For this review, take the finished solid that the model builds, in its own axes (mm). Face numbers are marked on the shaded views. A direction names the side the tool comes from. Coordinates: 2 decimals unless noted, no trailing zeros. Write each loop counter-clockwise with the first axis right and the second up, starting at its lowest first coordinate (ties: lowest second). Pieces come first, ordered by that corner, then holes.
1) To check wall thickness, follow line 1 along X through (y, z) = (-63, 0); line 2 along Z through (x, y) = (23, -10.5). State the ranges of each line that lie inside material, in increasing order.
2) For the marked faces 1, 2 and 3, list the 3-axis set-ups (+Z, -Z, +X, -X, +Y, -Y) from which the entire face can be reached by the end or side of a thin tool; tool diameter is ignored.
3) We need section A-A on z = 54.5. Write out the cut boundary in (x, y).
4) Insertion check: P1, Ø3, axis at x = 0, y = 53, coming from the -Z side; P2, Ø1, axis at y = 11.5, z = 33, coming from the +X side; P3, Ø1, axis at y = -54.5, z = 19.5, coming from the +X side. Each pin has a flat end and moves straight along its axis. Give the tip position at first contact, or say it passes through.
5) Mouldability with a two-part tool opening along Z and no side actions: class the marked faces 4, 5, 6 and 7 as pulls with the +Z half, pulls with the -Z half, needs draft (parallel to the pull), parting line crosses it, or undercut.
Autodesk Inventor part; units mm, degrees
ref_plane "YZ Plane" through (0, 0, 0) normal (1, 0, 0) x (0, 1, 0)
ref_plane "XZ Plane" through (0, 0, 0) normal (0, 1, 0) x (-1, 0, 0)
ref_plane "XY Plane" through (0, 0, 0) normal (0, 0, 1) x (1, 0, 0)
sketch "Sketch_1" plane through (0, 0, 0) normal (1, 0, 0) x (0, 1, 0)
  line L0 (61.0702, 0) -> (61.0702, -13.6667)
  line L1 (61.0702, -13.6667) -> (58.5831, -20.5)
  line L2 (58.5831, -20.5) -> (40.0529, -20.5)
  line L3 (40.0529, -20.5) -> (38.848, -17.1896)
  line L4 (38.848, -17.1896) -> (38.848, -13.6667)
  line L5 (-38.848, -13.6667) -> (-38.848, -17.1896)
  line L6 (-38.848, -17.1896) -> (-40.0529, -20.5)
  line L7 (-40.0529, -20.5) -> (-58.5831, -20.5)
  line L8 (-58.5831, -20.5) -> (-61.0702, -13.6667)
  line L9 (-61.0702, -13.6667) -> (-61.0702, 0)
  line L10 (-61.0702, 0) -> (61.0702, 0)
  line L11 (-40.0529, -20.5) -> (0, -20.5) construction
  line L12 (0, -20.5) -> (0, -30.1874) construction
  line L13 (-59.3111, -20.5) -> (-42.0529, -20.5)
  line L14 (-42.0529, -20.5) -> (-42.0529, -18.5)
  line L15 (-42.0529, -18.5) -> (-59.3111, -18.5)
  line L16 (-59.3111, -18.5) -> (-59.3111, -20.5)
  line L17 (42.0529, -20.5) -> (59.3111, -20.5)
  line L18 (59.3111, -20.5) -> (59.3111, -18.5)
  line L19 (59.3111, -18.5) -> (42.0529, -18.5)
  line L20 (42.0529, -18.5) -> (42.0529, -20.5)
  line L21 (-38.848, -13.6667) -> (38.848, -13.6667)
  point P0 (0, 0)
  point P1 (0, 0)
  point P2 (-49.318, -20.5)
  point P3 (50.682, -20.5)
  point P4 (0, 0)
  dimension "dimE" = 41
  dimension "d22" = 20.5
  dimension "d23" = 6.8333
  dimension "d24" = 20
  dimension "d27" = 22.2222
  dimension "d28" = 22.2222
  dimension "d52" = 20
  dimension "d53" = 2
  dimension "d54" = 2
  dimension "d55" = 2
  dimension "dimZ" = 100
revolve "Revolution1" add sketch "Sketch_1" angle 360 about axis through (0, -61.0702, 0) along (0, 1, 0) contours L0 L1 L19 L20 L2 L3 L4 L21 L5 L6 L7 L14 L15 L8 L9 L10 | L1 L2 L20 L19 | L15 L14 L7 L8 | L8 L13 L16
sketch "Sketch11" plane through (0, 0, 0) normal (0, 0, 1) x (1, 0, 0)
  line L0 (-23.848, 23.848) -> (23.848, 23.848)
  line L1 (23.848, 23.848) -> (23.848, -23.848)
  line L2 (23.848, -23.848) -> (-23.848, -23.848)
  line L3 (-23.848, -23.848) -> (-23.848, 23.848)
  line L4 (23.848, -23.848) -> (-23.848, 23.848)
  line L5 (17.1896, 38.848) -> (-17.1896, 38.848)
  point P0 (0, 0)
  point P1 (0, 0)
  point P2 (0, 0)
  dimension "d71" = 15
extrude "Extrusion6" add sketch "Sketch11" along normal blind 34
sketch "Sketch_2" plane through (0, 0, 0) normal (1, 0, 0) x (0, 1, 0)
  line L0 (0, 34) -> (23.848, 34)
  line L1 (23.848, 34) -> (23.848, 56.2222)
  line L2 (23.848, 56.2222) -> (0, 56.2222)
  line L3 (0, 56.2222) -> (0, 34)
  line L4 (0, 56.2222) -> (34.9591, 56.2222)
  line L5 (34.9591, 56.2222) -> (34.9591, 129)
  line L6 (34.9591, 129) -> (0, 129)
  line L7 (0, 129) -> (0, 56.2222)
  line L8 (-33.3229, 0) -> (54.4515, 0)
  line L9 (-90.3, 0) -> (90.3, 0)
  line L10 (0, -319.9275) -> (0, 424.6014)
  point P0 (10.5643, 0)
  dimension "d67" = 22.2222
  dimension "d68" = 129
  dimension "d70" = 11.1111
revolve "Revolution2" add sketch "Sketch_2" angle 360 about axis through (0, 0, 129) along (0, 0, -1)
fillet "Fillet1" radius 6.7 4 edges at (-23.848, 23.848, 17) (-23.848, -23.848, 17) (23.848, -23.848, 17) (23.848, 23.848, 17)
sketch "Sketch_7" plane through (0, 0, 0) normal (1, 0, 0) x (0, 1, 0)
  line L0 (-64.5, 12.5) -> (64.5, 12.5)
  line L1 (48.5126, 0) -> (-48.5126, 0)
  line L2 (-64.5, 12.5) -> (-64.5, 10)
  line L3 (-64.5, 10) -> (64.5, 10)
  line L4 (64.5, 10) -> (64.5, 12.5)
  line L5 (0, 0.4963) -> (0, 17.9963)
  point P0 (0, 0)
  point P1 (0, 0)
  point P2 (0, 10)
  point P3 (0, 0)
  dimension "dimH" = 129
  dimension "dimD" = 20
  dimension "dimD2" = 25
revolve "Revolution3" add sketch "Sketch_7" angle 360 about axis through (0, 48.5126, 0) along (0, -1, 0)
extrude "Extrusion8" cut sketch "Sketch_1" along normal mid plane 2.7333 contours L18 L17 L1 | L1 L2 L20 L19 | L15 L14 L7 L8 | L8 L13 L16
pattern_circular "Circular Pattern1" count 6 over 360 about axis through (0, 32.25, 0) along (0, -1, 0) of "Extrusion8"
equation "\"d23\" = 0.333333 * d22"
equation "\"d27\" = 0.222222 * dimZ"
equation "\"d28\" = d27"
equation "\"d35\" = 0.1 * dimC"
equation "\"d47\" = 0.0666667 * dimE"
properties part number "DIAPHRAGM VALVE PNEUMATIC GLUED DN15" material "PVC"
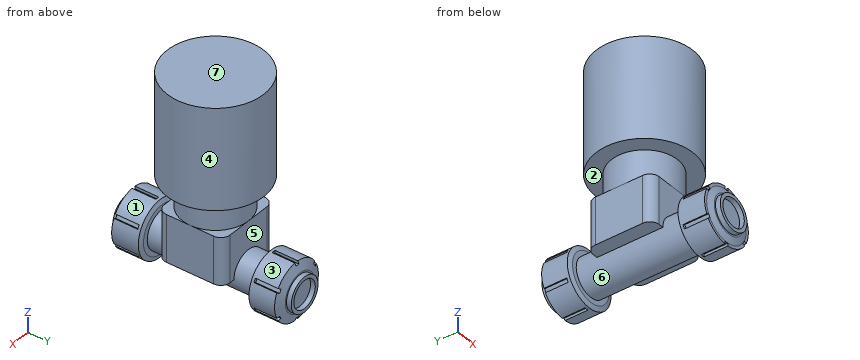
Result:
1. line 1: x = -12.5 to -10, 10 to 12.5
1. line 2: z = 0 to 34, 56.22 to 129
2. face 1: -Y
2. face 2: none
2. face 3: +Y
3. outline: circle Ø47.7 at (0, 0)
4. P1: stops at z = -20.45
4. P2: stops at x = 23.85
4. P3: stops at x = 7.7
5. face 4: needs draft
5. face 5: undercut
5. face 6: undercut
5. face 7: pulls with the +Z half
